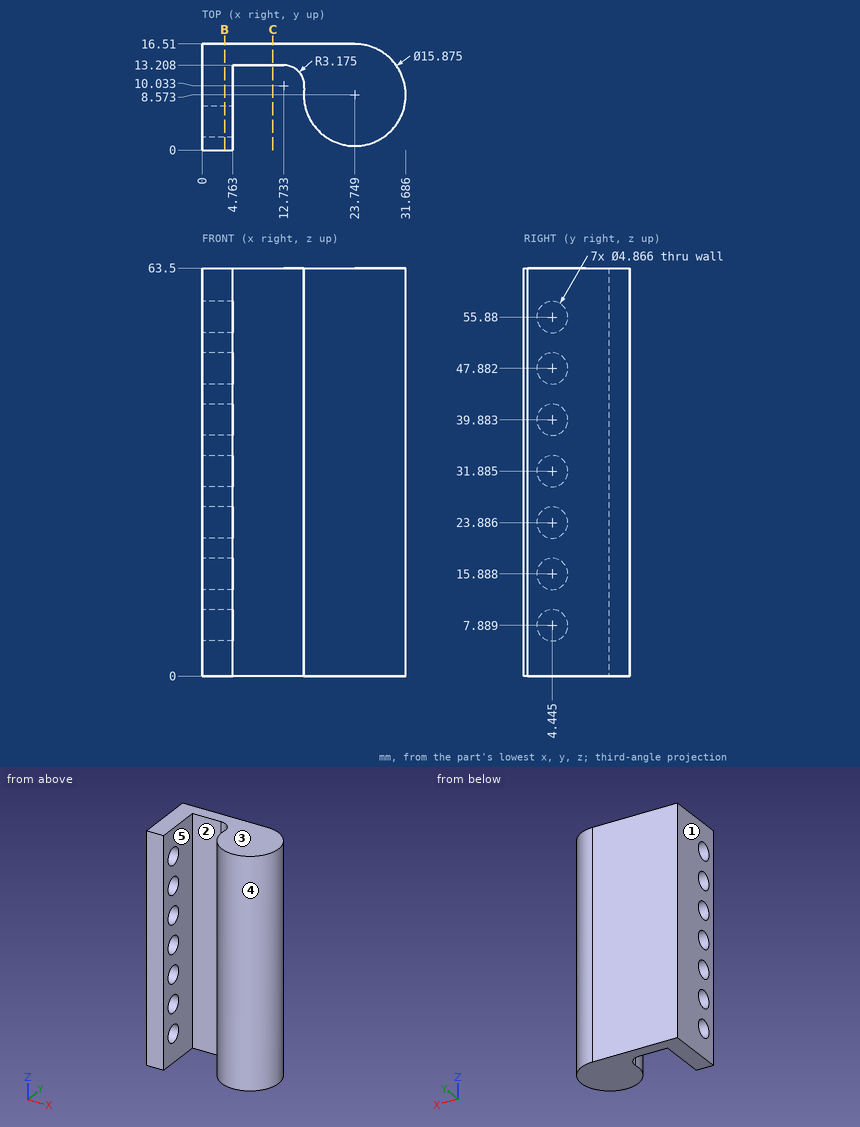
Job drawing, mm, ordinate dimensions from the low corner. One solid piece. A direction names the side the tool comes from. Round coordinates to 2 decimals unless told otherwise and drop trailing zeros. Order: outer loops, then holes, each group sorted by start corner. A loop starts at its lowest first (then second) coordinate and runs counter-clockwise, first axis right, second up. Notation, with made-up numbers: (7, -28) -> (37, -28) arc R29 ccw to (37, 6) -> close; hole circle Ø4 at (-7, 36). An arc over 180 degrees is marked (long way). Answer in a Markdown table with one row per item.
1) Which spindle directions (+Z, -Z, +X, -X, +Y, -Y) get a long thin tool onto all of the face, cutting with end or side? Do the marked faces 4 and 5. Say none if no direction does.
Values:
| item | result |
|---|---|
| face 4 | +Z, -Z |
| face 5 | +Z, -Z, -Y |
2) Pin check, flat tips, straight feed: P1, Ø4.5, axis at y = 4.445, z = 55.88, coming from the -X side; P2, Ø3, axis at y = 4.44, z = 23.89, coming from the -X side; P3, Ø3, axis at x = 19.5, z = 25, coming from the -Y side; P4, Ø8, axis at y = 4.44, z = 7.89, coming from the +X side (1 decimal). Stop position of each tip, or through.
Values:
| item | result |
|---|---|
| P1 | x = 16.04 |
| P2 | x = 16.26 |
| P3 | y = 1.13 |
| P4 | x = 31.7 |
3) Band-saw the part on B-B on x = 3.5. Give the cut face in (y, z) (1 decimal).
Values:
| item | result |
|---|---|
| outline | (0, 0) -> (16.5, 0) -> (16.5, 63.5) -> (0, 63.5) -> close; hole circle Ø4.9 at (4.4, 7.9); hole circle Ø4.9 at (4.4, 15.9); hole circle Ø4.9 at (4.4, 23.9); hole circle Ø4.9 at (4.4, 31.9); hole circle Ø4.9 at (4.4, 39.9); hole circle Ø4.9 at (4.4, 47.9); hole circle Ø4.9 at (4.4, 55.9) |
4) Wall check: L1, parallel to X at y = 8.5, z = 31.5; L2, parallel to X at y = 7.5, z = 15 (1 decimal); L3, parallel to Y at x = 6, z = 20. Give the ranges that are in metal, low to high.
Values:
| item | result |
|---|---|
| L1 | 0 to 4.76, 15.81 to 31.69 |
| L2 | 0 to 4.8, 15.9 to 31.6 |
| L3 | 13.21 to 16.51 |
5) Mould opens along X. For the marked faces 1, 2 and 3 say: released by +X, released by -X, zero draft, split by the parting line, or undercut.
Values:
| item | result |
|---|---|
| face 1 | released by -X |
| face 2 | undercut |
| face 3 | zero draft |
6) Band-saw the part on C-C on x = 11. Give the cut face in (y, z).
Values:
| item | result |
|---|---|
| outline | (13.21, 0) -> (16.51, 0) -> (16.51, 63.5) -> (13.21, 63.5) -> close |
